Source: CAD feature listing. Evaluate the final solid. Frame: model axes, mm. A direction names the side the tool comes from. Round coordinates to 2 decimals unless told otherwise and drop trailing zeros. Loops run counter-clockwise (first coordinate to the right, second up) from the corner with the lowest first, then second, coordinate; pieces in that order, holes last. Notation, with made-up numbers: M -20.5,27 L 6.5,27 A30 ccw 6.5,54 Z; hole C -5,-40 d5. An arc over 180 degrees is marked long. Answer as a JSON object with one key per item and string values.
Autodesk Inventor part; units mm, degrees
ref_plane "YZ Plane" through (0, 0, 0) normal (1, 0, 0) x (0, 1, 0)
ref_plane "XZ Plane" through (0, 0, 0) normal (0, 1, 0) x (-1, 0, 0)
ref_plane "XY Plane" through (0, 0, 0) normal (0, 0, 1) x (1, 0, 0)
sketch "Sketch1" plane through (-52, 0, -35) normal (0, -1, 0) x (1, 0, 0)
  line L0 (0, 70) -> (104, 70)
  line L1 (104, 70) -> (112, 62)
  line L2 (112, 62) -> (112, 8)
  line L3 (112, 8) -> (104, 0)
  line L4 (104, 0) -> (0, 0)
  line L5 (0, 0) -> (-8, 8)
  line L6 (-8, 8) -> (-8, 62)
  line L7 (-8, 62) -> (0, 70)
  circle A0 centre (27, 10) radius 5.5
  circle A1 centre (27, 60) radius 5.5
  circle A2 centre (77, 60) radius 5.5
  circle A3 centre (77, 10) radius 5.5
  circle A4 centre (52, 60) radius 2
  arc A5 (50, 6) -> (54, 6) centre (52, 6) ccw
  line L8 (54, 6) -> (54, 14)
  arc A6 (54, 14) -> (50, 14) centre (52, 14) ccw
  line L9 (50, 14) -> (50, 6)
  circle A7 centre (77, 35) radius 2
  arc A8 (23, 37) -> (23, 33) centre (23, 35) ccw
  line L10 (23, 33) -> (31, 33)
  arc A9 (31, 33) -> (31, 37) centre (31, 35) ccw
  line L11 (31, 37) -> (23, 37)
  arc A10 (66.5, 62.5) -> (62.5, 62.5) centre (64.5, 62.5) ccw
  line L12 (62.5, 62.5) -> (62.5, 7.5)
  arc A11 (62.5, 7.5) -> (66.5, 7.5) centre (64.5, 7.5) ccw
  line L13 (66.5, 7.5) -> (66.5, 62.5)
  arc A12 (105.3, 62) -> (98.7, 62) centre (102, 62) ccw
  line L14 (98.7, 62) -> (98.7, 58)
  arc A13 (98.7, 58) -> (105.3, 58) centre (102, 58) ccw
  line L15 (105.3, 58) -> (105.3, 62)
  arc A14 (5.3, 62) -> (-1.3, 62) centre (2, 62) ccw
  line L16 (-1.3, 62) -> (-1.3, 58)
  arc A15 (-1.3, 58) -> (5.3, 58) centre (2, 58) ccw
  line L17 (5.3, 58) -> (5.3, 62)
  arc A16 (-1.3, 8) -> (5.3, 8) centre (2, 8) ccw
  line L18 (5.3, 8) -> (5.3, 12)
  arc A17 (5.3, 12) -> (-1.3, 12) centre (2, 12) ccw
  line L19 (-1.3, 12) -> (-1.3, 8)
  arc A18 (98.7, 8) -> (105.3, 8) centre (102, 8) ccw
  line L20 (105.3, 8) -> (105.3, 12)
  arc A19 (105.3, 12) -> (98.7, 12) centre (102, 12) ccw
  line L21 (98.7, 12) -> (98.7, 8)
  point P0 (52, 35)
extrude "Extrusion1" add sketch "Sketch1" against normal up to surface (15 mm away) contours L0 L1 L2 L3 L4 L5 L6 L7 | A0 | A1 | A2 | A3 | A4 | L9 A6 L8 A5 | A7 | L11 A9 L10 A8 | L13 A11 L12 A10 | L15 A13 L14 A12 | L17 A15 L16 A14 | L19 A17 L18 A16 | L21 A19 L20 A18
hole "M6CBore" at (25, 0, -25) at (-25, 0, -25) at (-25, 0, 25) at (25, 0, 25) direction (0, 1, 0) diameter 6.6 end through all counterbore diameter 11 counterbore depth 6.8
extrude "M6ClearanceSlots" cut sketch "Sketch1" against normal through all contours L15 A13 L14 A12 | L17 A15 L16 A14 | L19 A17 L18 A16 | L21 A19 L20 A18
sketch "Sketch2" plane through (-52, 15, -35) normal (0, 1, 0) x (1, 0, 0)
  line L0 (52, -14) -> (52, -6) construction
  line L1 (54, -14) -> (54, -6)
  line L2 (50, -6) -> (50, -14)
  arc A0 (50, -14) -> (54, -14) centre (52, -14) ccw
  arc A1 (54, -6) -> (50, -6) centre (52, -6) ccw
  point P0 (52, -35)
  point P1 (52, -60)
  point P2 (52, -10)
  dimension "d11" = 4
hole "Hole2" at (0, 15, 25) direction (0, -1, 0) diameter 4 depth 8 tip angle 118
extrude "Extrusion3" cut sketch "Sketch2" against normal blind 8
properties part number "FAB-P0001" material "SolidWorks Materials|6061-T6 (SS)"
Item 1: Line query: probe 1 along X at (y, z) = (11.5, 25); probe 2 along X at (y, z) = (1.5, -25); probe 3 along Z at (x, y) = (-23.5, 3). Output: solid intervals per line, ascending. Write a range as from..to.
Answer sheet:
{"probe 1": "x = -60..-53.3, -46.7..-28.3, -21.7..-2, 2..21.7, 28.3..46.7, 53.3..60", "probe 2": "x = -60..-53.3, -46.7..-30.5, -19.5..19.5, 30.5..46.7, 53.3..60", "probe 3": "z = -35..-30.29, -19.71..19.71, 30.29..35"}
Item 2: Section B-B on x = 50. Return the cut outline in (y, z), then the cut area to 3 significant figures.
Answer sheet:
{"outline": "M 0,-35 L 15,-35 L 15,-30.3 L 0,-30.3 Z; M 0,-19.7 L 15,-19.7 L 15,19.7 L 0,19.7 Z; M 0,30.3 L 15,30.3 L 15,35 L 0,35 Z", "area": "732 mm²"}
Item 3: Access query for faces 1 (the cylindrical face through (-26.652, 3.448, 19.754)), 2 (the cylindrical face through (-50.1, 7.4, 19.7)), 3 (the flat face through (-56, 7, 31)). Directions: +Z, -Z, +X, -X, +Y, -Y. A direction counts if a zero-diameter tool reaches every point of the face in a straight line with its end or side. Return the directions, or none.
Answer sheet:
{"face 1": "-Y", "face 2": "+Y, -Y", "face 3": "+Z, -X, +Y, -Y"}
Item 4: Section A-A on x = 25. Return the cut outline in (y, z).
Answer sheet:
{"outline": "M 0,-35 L 15,-35 L 15,-28.3 L 6.8,-28.3 L 6.8,-30.5 L 0,-30.5 Z; M 0,-19.5 L 6.8,-19.5 L 6.8,-21.7 L 15,-21.7 L 15,21.7 L 6.8,21.7 L 6.8,19.5 L 0,19.5 Z; M 0,30.5 L 6.8,30.5 L 6.8,28.3 L 15,28.3 L 15,35 L 0,35 Z"}
Item 5: Pull-direction query (Z, two-part tool) for faces 4 (the conical face through (0.104, 6.007, 25.331)), 5 (the flat face through (-56, 7, -31)), 6 (the flat face through (0, 7, -25)), 7 (the flat face through (56, 7, 31)); classes: pulls with the +Z half, pulls with the -Z half, needs draft (parallel to the pull), parting line crosses it, or undercut.
Answer sheet:
{"face 4": "undercut", "face 5": "pulls with the -Z half", "face 6": "undercut", "face 7": "pulls with the +Z half"}
Item 6: Contact query for flat-ended pins moving along their axis: pin 1 Ø5.5 at (x, z) = (-22.5, 25.5) entering from -Y; pin 2 Ø4 at (x, z) = (25, 25) entering from -Y. Output: stop coordinate, or through.
Answer sheet:
{"pin 1": "stops at y = 6.8", "pin 2": "passes through"}
